The listing builds one solid part. Answer for the finished solid, in the listing's coordinates (mm). Round coordinates to 2 decimals unless told otherwise and drop trailing zeros. Write each loop counter-clockwise with the first axis right and the second up, starting at its lowest first coordinate (ties: lowest second). Pieces come first, ordered by that corner, then holes.
(1) A cutting plane is placed at D-D, the plane x = -2.2. Give the vertices of the cut face in (y, z), and give its area (3 significant figures).
(2) The mould has two halves that part along Y. Classify faces 1 (the face through (1, 0, 0.2)), 2 (the face through (0, -2, 0)): +Y half, -Y half, draft (parallel to the pull), parting line (faces both ways), or undercut.
(3) Find the intervals of material crossed by probe 1 along Y at (x, z) = (0, 0.15); probe 2 along Z at (x, y) = (0.2, -1); probe 3 along X at (y, z) = (2.15, -0.05), in increasing order.
(4) A cutting plane is placed at C-C, the plane z = -3.05. Give the vertices of the cut face in (x, y).
(5) This flat-tipped pin is pushed along its axis until it touches: pin 1 Ø1.5 at (y, z) = (-2, -4) entering from +X. Where does it stop, or does it pass through?
from build123d import *

# Parameters (mm, degrees)
SKETCH_1_R          = 2.5
EXTRUDE_1_DEPTH     = 0.2
EXTRUDE_START       = 0.2
SKETCH_3_R          = 2.5
SKETCH_3_R_2        = 2.4
EXTRUDE_2_DEPTH     = 0.2
SKETCH_4_R          = 1.75
SKETCH_4_R_2        = 1.65
CUT_EXTRUDE_1_DEPTH = 0.1
SKETCH_5_R          = 0.3
SKETCH_5_R_2        = 0.25
EXTRUDE_3_DEPTH     = 5.5
FILLET_1_R          = 0.03
CUT_EXTRUDE_START   = -5.5
SKETCH_11_R         = 0.25
CUT_EXTRUDE_3_DEPTH = 5.5


with BuildPart() as part:
    # 스케치1 → 보스-돌출1 (new body)
    with BuildSketch(Plane.XY):
        Circle(SKETCH_1_R)
    extrude(amount=EXTRUDE_1_DEPTH)

    # 스케치3 → 보스-돌출2 (add)
    with BuildSketch(Plane(origin=(0, 0, 0), x_dir=(-1, 0, 0), z_dir=(0, 0, -1)).offset(EXTRUDE_START)):
        Circle(SKETCH_3_R)
        Circle(SKETCH_3_R_2, mode=Mode.SUBTRACT)
    extrude(amount=-EXTRUDE_2_DEPTH)

    # 스케치4 → 컷-돌출1 (cut)
    with BuildSketch(Plane(origin=(0, 0, 0), x_dir=(-1, 0, 0), z_dir=(0, 0, -1))):
        Circle(SKETCH_4_R)
        Circle(SKETCH_4_R_2, mode=Mode.SUBTRACT)
    extrude(amount=-CUT_EXTRUDE_1_DEPTH, mode=Mode.SUBTRACT)

    # 스케치5 → 보스-돌출3 (add)
    with BuildSketch(Plane(origin=(0, 0, 0), x_dir=(-1, 0, 0), z_dir=(0, 0, -1))):
        with Locations(Location((0, 0, 0), (0, 0, 180))):
            Circle(SKETCH_5_R)
        Circle(SKETCH_5_R_2, mode=Mode.SUBTRACT)
    extrude(amount=EXTRUDE_3_DEPTH)

    # 스케치7 → 회전1 (revolve)
    with BuildSketch(Plane(origin=(0, 0, 0), x_dir=(1, 0, 0), z_dir=(0, 1, 0))):
        Polygon((0.3, 0), (0.3, 0.6), (0.365, 0.6), (0.5, 0), align=None)
    revolve(axis=Axis((0, 0, 0), (0, 0, -1)))

    # 필렛1
    fillet_1_edges = [part.edges().sort_by_distance(p)[0] for p in [
        (-0.365, 0, -0.6),
    ]]
    fillet(fillet_1_edges, radius=FILLET_1_R)

    # 스케치11 → 컷-돌출3 (cut)
    with BuildSketch(Plane(origin=(0, 0, 0), x_dir=(-1, 0, 0), z_dir=(0, 0, -1)).offset(CUT_EXTRUDE_START)):
        with Locations(Location((0, 0, 0), (0, 0, 180))):
            Circle(SKETCH_11_R)
    extrude(amount=CUT_EXTRUDE_3_DEPTH, mode=Mode.SUBTRACT)


solid = part.part
Solutions:
1. outline: (-1.19, -0.2) - (-0.96, -0.2) - (-0.96, 0) - (0.96, 0) - (0.96, -0.2) - (1.19, -0.2) - (1.19, 0.2) - (-1.19, 0.2) - close
1. area: 0.566 mm2
2. face 1: draft
2. face 2: undercut
3. probe 1: y = -2.5 to -0.25, 0.25 to 2.5
3. probe 2: z = 0 to 0.2
3. probe 3: x = -1.28 to -1.07, 1.07 to 1.28
4. outline: circle Ø0.6 at (0, 0); hole circle Ø0.5 at (0, 0)
5. pin 1: passes through
